Could you check a few things on this model? Use its own coordinates, in mm. A direction names the side the tool comes from. Round coordinates to 2 decimals unless told otherwise and drop trailing zeros. Loops run counter-clockwise (first coordinate to the right, second up) from the corner with the lowest first, then second, coordinate; pieces in that order, holes last. Notation, with made-up numbers: (66, -35) -> (112, -35) arc R21 ccw to (112, -18) -> close; hole circle Ø8 at (34, 84.25). An arc over 180 degrees is marked (long way). One line per item, written item: value.
```python
from build123d import *


with BuildPart() as part:
    # Sketch1 → Revolve1 (revolve)
    with BuildSketch(Plane.XY):
        with BuildLine():
            Line((116.957401038, 12.446), (21.359317213, 32.766))
            Line((21.359317213, 32.766), (15.009317213, 32.766))
            Line((15.009317213, 32.766), (0, 6.7691))
            Line((0, 6.7691), (0, 0.4191))
            Line((0, 0.4191), (9.525, 0.4191))
            Line((9.525, 0.4191), (9.525, -3.556))
            Line((9.525, -3.556), (25.944743879, -3.556))
            ThreePointArc((25.944743879, -3.556), (28.374783674, -3.072635031), (30.434871939, -1.696128061))
            Line((30.434871939, -1.696128061), (36.240128061, 4.109128061))
            ThreePointArc((36.240128061, 4.109128061), (38.300216326, 5.485635031), (40.730256121, 5.969))
            Line((40.730256121, 5.969), (116.957401038, 5.969))
            Line((116.957401038, 5.969), (116.957401038, 12.446))
        make_face()
    revolve(axis=Axis((0, 50.546, 0), (1, 0, 0)))


solid = part.part
```
Item 1: Will these pins go through, and if not, where does the flat tip stop? pin 1 Ø10 at (x, z) = (62.5, -12) entering from +Y; pin 2 Ø12 at (x, y) = (79.5, 57.5) entering from +Z; pin 3 Ø6 at (x, z) = (74, -9.5) entering from -Y; pin 4 Ø21.5 at (y, z) = (50.546, 0) entering from +X.
Output:
pin 1: stops at y = 94.57
pin 2: stops at z = 44.57
pin 3: stops at y = 6.45
pin 4: passes through
Item 2: If we mould it in two halves opening along Y, with no side actions, what happens to faces 4 (the face through (35.958, 60.674, 45.608)), 5 (the face through (14.07, 69.933, -0.853)), 6 (the face through (9.525, 66, 48))? For each: released by +Y, released by -Y, zero draft, split by the parting line, or undercut.
Output:
face 4: split by the parting line
face 5: undercut
face 6: zero draft
Item 3: If we section it at A-A on z = 0: List the corners of the cut face in (x, y) for me (3 decimals), plus the area to 3 significant figures.
Output:
outline: (0, 0.419) -> (9.525, 0.419) -> (9.525, -3.556) -> (25.945, -3.556) arc R6.35 ccw to (30.435, -1.696) -> (36.24, 4.109) arc R6.35 cw to (40.73, 5.969) -> (116.957, 5.969) -> (116.957, 12.446) -> (21.359, 32.766) -> (15.009, 32.766) -> (0, 6.769) -> close; (0, 94.323) -> (15.009, 68.326) -> (21.359, 68.326) -> (116.957, 88.646) -> (116.957, 95.123) -> (40.73, 95.123) arc R6.35 cw to (36.24, 96.983) -> (30.435, 102.788) arc R6.35 ccw to (25.945, 104.648) -> (9.525, 104.648) -> (9.525, 100.673) -> (0, 100.673) -> close
area: 4,490 mm²
Item 4: I need wall thicknesses on line 1 (Y direction, x = 18, z = 0); line 2 (Z direction, x = 27, y = 64); line 3 (Y direction, x = 20.5, z = 16). Which ranges of each line are inside material? Lowest first, please. Write a range as from..to.
Output:
line 1: y = -3.56..32.77, 68.33..104.65
line 2: z = -52.31..-13.39, 13.39..52.31
line 3: y = -1.14..42.79, 58.3..102.23
Item 5: If we section it at C-C on x = 47.5: List the corners of the cut face in (y, z) for me, plus the area to 3 significant figures.
Output:
outline: circle Ø89.15 at (50.55, 0); hole circle Ø46.67 at (50.55, 0)
area: 4,530 mm²
Item 6: For faces 1 (the face through (79.377, 8.027, -13.39)), 2 (the face through (4.829, 90.325, 30.501)), 3 (the face through (0, 50, 44)), which set-ups out of +Z, -Z, +X, -X, +Y, -Y let a thin tool reach every point of the face, with its end or its side?
Output:
face 1: +X
face 2: -X
face 3: +Z, -Z, -X, +Y, -Y
Item 7: If we section it at B-B on x = 72: List the corners of the cut face in (y, z) for me.
Output:
outline: circle Ø89.15 at (50.55, 0); hole circle Ø57.09 at (50.55, 0)
